Build history of the part. All positions in model axes, mm. A direction names the side the tool comes from. Round coordinates to 2 decimals unless told otherwise and drop trailing zeros. Write each loop counter-clockwise with the first axis right and the second up, starting at its lowest first coordinate (ties: lowest second). Pieces come first, ordered by that corner, then holes. Notation, with made-up numbers: (89, 85) -> (97, 85) arc R11 cw to (97, 100) -> close; hole circle Ø11 at (72, 67). An arc over 180 degrees is marked (long way). Answer in a Markdown table with one row per item.
```python
from build123d import *

# Parameters (mm, degrees)
EXTRUDE_2_DEPTH          = 3
SKETCH_2_R               = 1.25
CUT_EXTRUDE_1_DEPTH      = 4
PATTERN_CIRCULAR_1_COUNT = 4
EXTRUDE_3_DEPTH          = 0.75
SKETCH_4_W               = 2.5
SKETCH_4_H               = 2
EXTRUDE_5_DEPTH          = 3
PATTERN_LINEAR_1_COUNT   = 2
PATTERN_LINEAR_1_PITCH   = 35
SKETCH_5_W               = 2
SKETCH_5_H               = 2.5
EXTRUDE_6_DEPTH          = 3
PATTERN_LINEAR_2_COUNT   = 2
PATTERN_LINEAR_2_PITCH   = 33.5


with BuildPart() as part:
    # 草图1 → 凸台-拉伸2 (new body)
    with BuildSketch(Plane.XY):
        with BuildLine():
            Line((-5.25, -16), (-5, -16))
            Line((-5, -16), (0, -16))
            Line((0, -16), (5, -16))
            Line((5, -16), (5.25, -16))
            ThreePointArc((5.25, -16), (8.178932188, -8.928932188), (15.25, -6))
            Line((15.25, -6), (15.25, -5))
            Line((15.25, -5), (15.25, 0))
            Line((15.25, 0), (15.25, 5))
            Line((15.25, 5), (15.25, 6))
            ThreePointArc((15.25, 6), (8.178932188, 8.928932188), (5.25, 16))
            Line((5.25, 16), (5, 16))
            Line((5, 16), (0, 16))
            Line((0, 16), (-5, 16))
            Line((-5, 16), (-5.25, 16))
            ThreePointArc((-5.25, 16), (-8.178932188, 8.928932188), (-15.25, 6))
            Line((-15.25, 6), (-15.25, 5))
            Line((-15.25, 5), (-15.25, 0))
            Line((-15.25, 0), (-15.25, -5))
            Line((-15.25, -5), (-15.25, -6))
            ThreePointArc((-15.25, -6), (-8.178932188, -8.928932188), (-5.25, -16))
        make_face()
        Polygon((-1.25, -11), (-1.25, -4.5), (1.25, -4.5), (1.25, -11), (2.25, -11), (2.25, -13), (0, -13), (-2.25, -13), (-2.25, -11), align=None, mode=Mode.SUBTRACT)
        Polygon((-11, -2.25), (-13, -2.25), (-13, 0), (-13, 2.25), (-11, 2.25), (-11, 1.25), (-4.5, 1.25), (-4.5, -1.25), (-11, -1.25), align=None, mode=Mode.SUBTRACT)
        Polygon((4.5, -1.25), (4.5, 1.25), (11, 1.25), (11, 2.25), (13, 2.25), (13, 0), (13, -2.25), (11, -2.25), (11, -1.25), align=None, mode=Mode.SUBTRACT)
        Polygon((-2.25, 11), (-2.25, 13), (0, 13), (2.25, 13), (2.25, 11), (1.25, 11), (1.25, 4.5), (-1.25, 4.5), (-1.25, 11), align=None, mode=Mode.SUBTRACT)
    extrude(amount=EXTRUDE_2_DEPTH)

    # 草图2 → 切除-拉伸1 (cut)
    with BuildSketch(Plane(origin=(0, 16, 0), x_dir=(1, 0, 0), z_dir=(0, 1, 0))):
        with Locations((0, -1.5)):
            Circle(SKETCH_2_R)
    cut_extrude_1 = extrude(amount=-CUT_EXTRUDE_1_DEPTH, mode=Mode.SUBTRACT)

    # 阵列(圆周)1: 切除-拉伸1 ×4 about axis
    pattern_circular_1_axis = Axis((0, 0, 3), (0, 0, 1))
    for i in range(1, PATTERN_CIRCULAR_1_COUNT):
        add(cut_extrude_1.rotate(pattern_circular_1_axis, i * 360 / PATTERN_CIRCULAR_1_COUNT), mode=Mode.SUBTRACT)

    # 草图3 → 凸台-拉伸3 (add)
    with BuildSketch(Plane.XY.offset(3)):
        Polygon((1, 0.025113601), (0, 0), (0, 2), align=None)
        Polygon((-1, -0.025113601), (0, 2), (0, 0), align=None)
        Polygon((-1, -0.025113601), (0, 0), (0, -2), align=None)
        Polygon((1, 0.025113601), (0, -2), (0, 0), align=None)
    extrude(amount=EXTRUDE_3_DEPTH)

    # 草图4 → 凸台-拉伸5 (add)
    with BuildSketch(Plane(origin=(0, 16, 0), x_dir=(1, 0, 0), z_dir=(0, 1, 0))):
        with Locations((3.75, -1.5)):
            Rectangle(SKETCH_4_W, SKETCH_4_H)
        with Locations((-3.75, -1.5)):
            Rectangle(SKETCH_4_W, SKETCH_4_H)
    extrude_5 = extrude(amount=EXTRUDE_5_DEPTH)

    # 阵列(线性)1: 凸台-拉伸5 ×2
    with Locations(*[(0, -i * PATTERN_LINEAR_1_PITCH, 0) for i in range(1, PATTERN_LINEAR_1_COUNT)]):
        add(extrude_5)

    # 草图5 → 凸台-拉伸6 (add)
    with BuildSketch(Plane(origin=(15.25, 0, 0), x_dir=(0, 0, -1), z_dir=(1, 0, 0))):
        with Locations((-1.5, 3.75)):
            Rectangle(SKETCH_5_W, SKETCH_5_H)
        with Locations((-1.5, -3.699772798)):
            Rectangle(SKETCH_5_W, SKETCH_5_H)
    extrude_6 = extrude(amount=EXTRUDE_6_DEPTH)

    # 阵列(线性)2: 凸台-拉伸6 ×2
    with Locations(*[(-i * PATTERN_LINEAR_2_PITCH, 0, 0) for i in range(1, PATTERN_LINEAR_2_COUNT)]):
        add(extrude_6)


solid = part.part
```
Q1. Two-plate mould, pull along X, no slides. Class faces 1 (the flat face through (-1.25, 8, 1)), 2 (the flat face through (-18.25, 4, 2)), 3 (the flat face through (4, 17, 0.5)), 4 (the flat face through (18.25, -4, 2)): released by +X, released by -X, zero draft, split by the parting line, or undercut.
A:
| item | result |
|---|---|
| face 1 | undercut |
| face 2 | released by -X |
| face 3 | zero draft |
| face 4 | released by +X |
Q2. Saw through at A-A on y = 8. Write the cut outline in (x, z), plus the area to 3 significant figures.
A:
| item | result |
|---|---|
| outline | (-9.25, 0) -> (-1.25, 0) -> (-1.25, 3) -> (-9.25, 3) -> close; (1.25, 0) -> (9.25, 0) -> (9.25, 3) -> (1.25, 3) -> close |
| area | 48.0 mm² |
Q3. Saw through at D-D on x = -14. Write the cut outline in (y, z), plus the area to 3 significant figures.
A:
| item | result |
|---|---|
| outline | (-6.08, 0) -> (6.08, 0) -> (6.08, 3) -> (-6.08, 3) -> close; hole circle Ø2.5 at (0, 1.5) |
| area | 31.6 mm² |
Q4. Saw through at B-B on x = 7. Write the cut outline in (y, z), plus the area to 3 significant figures.
A:
| item | result |
|---|---|
| outline | (-10.35, 0) -> (-1.25, 0) -> (-1.25, 3) -> (-10.35, 3) -> close; (1.25, 0) -> (10.35, 0) -> (10.35, 3) -> (1.25, 3) -> close |
| area | 54.6 mm² |
Q5. Saw through at C-C on x = -3. Write the cut outline in (y, z).
A:
| item | result |
|---|---|
| outline | (-19, 0.5) -> (-16, 0.5) -> (-16, 0) -> (16, 0) -> (16, 0.5) -> (19, 0.5) -> (19, 2.5) -> (16, 2.5) -> (16, 3) -> (-16, 3) -> (-16, 2.5) -> (-19, 2.5) -> close |
Q6. Wall check: line 1 (X direction, y = 2, z = 2.05); line 2 (X direction, y = 1, z = 0.4); line 3 (Z direction, x = -13.9, y = 0). Give the ranges that are in metal, low to high. Write a range as [from, to].
A:
| item | result |
|---|---|
| line 1 | [-15.25, -13], [-11, 11], [13, 15.25] |
| line 2 | [-15.25, -13], [-4.5, 4.5], [13, 15.25] |
| line 3 | [0, 0.25], [2.75, 3] |
Q7. Which spindle directions (+Z, -Z, +X, -X, +Y, -Y) get a long thin tool onto all of the face, cutting with end or side? Do faces 5 (the flat face through (17, -4.95, 2)), 6 (the flat face through (2.25, 12, 1)), 7 (the cylindrical face through (0.99, -14.52, 2.26)), 8 (the flat face through (-17, -2.45, 2)). Say none if no direction does.
A:
| item | result |
|---|---|
| face 5 | +Z, -Z, +X, -Y |
| face 6 | +Z, -Z |
| face 7 | -Y |
| face 8 | +Z, -Z, -X |
Q8. Drop flat-ended pins along their axis: P1, Ø2, axis at y = -18, z = 1.5, coming from the -X side; P2, Ø2, axis at y = 0, z = 1.5, coming from the +X side; P3, Ø2, axis at x = 12.5, z = 1.5, coming from the -Y side; P4, Ø3, axis at x = 16.5, y = 3, coming from the -Z side. Give the stop position or say it passes through.
A:
| item | result |
|---|---|
| P1 | x = -5 |
| P2 | x = 4.5 |
| P3 | y = -6.73 |
| P4 | z = 0 |
